Could you check a few things on this model? Use its own coordinates, in mm. A direction names the side the tool comes from. Round coordinates to 2 decimals unless told otherwise and drop trailing zeros. Write each loop counter-clockwise with the first axis right and the second up, starting at its lowest first coordinate (ties: lowest second). Pieces come first, ordered by that corner, then holes. Notation, with made-up numbers: (56.25, 32.5) -> (72.25, 32.5) arc R27 cw to (72.25, 61.5) -> close; hole circle Ø1 at (-7.75, 77). An arc over 180 degrees is marked (long way). Answer in a Markdown table with one row per item.
from build123d import *

# Parameters (mm, degrees)
SKETCH1_W           = 100
SKETCH1_H           = 100
BOSS_EXTRUDE1_DEPTH = 10
SKETCH6_W           = 40
SKETCH6_H           = 40
BOSS_EXTRUDE3_DEPTH = 34
SKETCH8_W           = 20
SKETCH8_H           = 10
CUT_EXTRUDE1_DEPTH  = 10
SKETCH9_W           = 20
SKETCH9_H           = 10
CUT_EXTRUDE2_DEPTH  = 10
SKETCH10_W          = 10
SKETCH10_H          = 12
CUT_EXTRUDE3_DEPTH  = 34


with BuildPart() as part:
    # Sketch1 → Boss-Extrude1 (new body)
    with BuildSketch(Plane(origin=(0, 0, 0), x_dir=(1, 0, 0), z_dir=(0, 1, 0))):
        Rectangle(SKETCH1_W, SKETCH1_H)
    extrude(amount=BOSS_EXTRUDE1_DEPTH)

    # Sketch6 → Boss-Extrude3 (add)
    with BuildSketch(Plane(origin=(0, 10, 0), x_dir=(1, 0, 0), z_dir=(0, 1, 0))):
        Rectangle(SKETCH6_W, SKETCH6_H)
    extrude(amount=BOSS_EXTRUDE3_DEPTH)

    # Sketch8 → Cut-Extrude1 (cut)
    with BuildSketch(Plane(origin=(0, 10, 0), x_dir=(1, 0, 0), z_dir=(0, 1, 0))):
        with Locations((-20, -45)):
            Rectangle(SKETCH8_W, SKETCH8_H)
    extrude(amount=-CUT_EXTRUDE1_DEPTH, mode=Mode.SUBTRACT)

    # Sketch9 → Cut-Extrude2 (cut)
    with BuildSketch(Plane(origin=(0, 10, 0), x_dir=(1, 0, 0), z_dir=(0, 1, 0))):
        with Locations((20, -45)):
            Rectangle(SKETCH9_W, SKETCH9_H)
    extrude(amount=-CUT_EXTRUDE2_DEPTH, mode=Mode.SUBTRACT)

    # Sketch10 → Cut-Extrude3 (cut)
    with BuildSketch(Plane(origin=(0, 44, 0), x_dir=(1, 0, 0), z_dir=(0, 1, 0))):
        with Locations((15, 0)):
            Rectangle(SKETCH10_W, SKETCH10_H)
        with Locations((-15, 0)):
            Rectangle(SKETCH10_W, SKETCH10_H)
    extrude(amount=-CUT_EXTRUDE3_DEPTH, mode=Mode.SUBTRACT)


solid = part.part
1) Imagine slicing it at D-D, the plane y = 39. Please give me the cut outline in (x, z).
Findings:
| item | result |
|---|---|
| outline | (-20, -20) -> (20, -20) -> (20, -6) -> (10, -6) -> (10, 6) -> (20, 6) -> (20, 20) -> (-20, 20) -> (-20, 6) -> (-10, 6) -> (-10, -6) -> (-20, -6) -> close |
2) Imagine slicing it at B-B, the plane y = 5. Please give me the cut outline in (x, z), plus the area to 3 significant figures.
Findings:
| item | result |
|---|---|
| outline | (-50, -50) -> (50, -50) -> (50, 50) -> (30, 50) -> (30, 40) -> (10, 40) -> (10, 50) -> (-10, 50) -> (-10, 40) -> (-30, 40) -> (-30, 50) -> (-50, 50) -> close |
| area | 9,600 mm^2 |
3) Thinking about a two-plate mould opening in Z: for faces 1 (the face through (20, 27, -13)), 2 (the face through (-10, 27, 0)), 3 (the face through (-40, 5, 50)), which applies, +Z half, -Z half, draft (parallel to the pull), parting line (faces both ways), or undercut?
Findings:
| item | result |
|---|---|
| face 1 | draft |
| face 2 | undercut |
| face 3 | +Z half |
4) For faces 4 (the face through (15, 27, 6)), 5 (the face through (-20, 27, 13)), 6 (the face through (0, 27, -20)), which set-ups out of +Z, -Z, +X, -X, +Y, -Y let a thin tool reach every point of the face, with its end or its side?
Findings:
| item | result |
|---|---|
| face 4 | +X, +Y |
| face 5 | +Z, -Z, -X, +Y |
| face 6 | -Z, +X, -X, +Y |
5) Imagine slicing it at C-C, the plane x = 28. Please give me the cut outline in (y, z), plus the area to 3 significant figures.
Findings:
| item | result |
|---|---|
| outline | (0, -50) -> (10, -50) -> (10, 40) -> (0, 40) -> close |
| area | 900 mm^2 |
6) For pin 1 (5 mm diameter, centred on x = -15.5, y = 33.5, fed in from +Z); pin 2 (1 mm diameter, centred on y = 32, z = 17, fed in from +X); pin 3 (7 mm diameter, centred on y = 27, z = 12, fed in from -X), each with a flat end and sliding along its axis, tell me the tip position at first contact or that it passes through.
Findings:
| item | result |
|---|---|
| pin 1 | stops at z = 20 |
| pin 2 | stops at x = 20 |
| pin 3 | stops at x = -20 |
7) Imagine slicing it at A-A, the plane z = -14. Please give me the cut outline in (x, y), plus the area to 3 significant figures.
Findings:
| item | result |
|---|---|
| outline | (-50, 0) -> (50, 0) -> (50, 10) -> (20, 10) -> (20, 44) -> (-20, 44) -> (-20, 10) -> (-50, 10) -> close |
| area | 2,360 mm^2 |
8) Please list where these lines run through material, in increasing order: line 1 (Z direction, x = -17.5, y = 28.5); line 2 (Y direction, x = -36.5, z = -2); line 3 (X direction, y = 34, z = 17).
Findings:
| item | result |
|---|---|
| line 1 | z = -20 to -6, 6 to 20 |
| line 2 | y = 0 to 10 |
| line 3 | x = -20 to 20 |
